from build123d import *

# Parameters (mm, degrees)
BOSS_EXTRUDE1_DEPTH = 10
CUT_EXTRUDE1_START  = -10
CUT_EXTRUDE1_DEPTH  = 10


with BuildPart() as part:
    # Sketch1 → Boss-Extrude1 (new body)
    with BuildSketch(Plane(origin=(0, 0, 0), x_dir=(1, 0, 0), z_dir=(0, 1, 0))):
        Polygon((-19.75, 34.208003449), (-39.5, 0), (-19.75, -34.208003449), (19.75, -34.208003449), (39.5, 0), (19.75, 34.208003449), align=None)
    extrude(amount=BOSS_EXTRUDE1_DEPTH)

    # Sketch7 → Revolve1 (revolve)
    with BuildSketch(Plane(origin=(0, 0, 0), x_dir=(0, 0, -1), z_dir=(1, 0, 0))):
        with BuildLine():
            Line((0, 10), (0, 50))
            Line((0, 50), (3.95, 50))
            Line((3.95, 50), (3.95, 27.320508076))
            ThreePointArc((3.95, 27.320508076), (6.629491924, 17.320508076), (13.95, 10))
            Line((13.95, 10), (0, 10))
        make_face()
    revolve(axis=Axis((0, 10, 0), (0, 1, 0)))

    # Sketch8 → Cut-Extrude1 (cut)
    with BuildSketch(Plane(origin=(0, 50, 0), x_dir=(1, 0, 0), z_dir=(0, 1, 0)).offset(CUT_EXTRUDE1_START)):
        with BuildLine():
            Line((-3.058185737, -2.5), (-3.058185737, 2.5))
            ThreePointArc((-3.058185737, 2.5), (-3.95, 0), (-3.058185737, -2.5))
        make_face()
    extrude(amount=CUT_EXTRUDE1_DEPTH, mode=Mode.SUBTRACT)


solid = part.part
Verification items for the finished model (mm, model axes). A direction names the side the tool comes from. Give positions to 0.01 mm unless a question says otherwise; leave off trailing zeros. Write each loop counter-clockwise with the first axis right and the second up, starting at its lowest first coordinate (ties: lowest second). Pieces come first, ordered by that corner, then holes. Notation, with made-up numbers: M -27,47.25 L 30,47.25 A32 cw 30,85.25 Z; hole C 83.25,-7 d5. An arc over 180 degrees is marked long. Put each result on its own line as item: value. Start each with the question number.
1. Scan lines: line 1 along Y through (x, z) = (23, -9.5); line 2 along X through (y, z) = (6, -27); line 3 along Z through (x, y) = (-31.5, 9.5). Record each from-to range of solid material in increasing order. Write a range as [from, to].
2. Section check C-C (z = 20.5). Record the cut outline in (x, y), and give its area (3 significant figures).
3. Section check D-D (x = 31.5). Record the cut outline in (y, z), and give its area (3 significant figures).
4. Go/stop test with flat-tipped pins: pin 1 Ø10 at (y, z) = (44.5, -4) entering from -X; pin 2 Ø1.5 at (y, z) = (43, 0.5) entering from -X. Record where each tip stops, or that it passes through.
5. Set-up check for faces 4 (the face through (17, 10, 0)), 5 (the face through (-3.058, 45, 0)), 6 (the face through (0, 5, 34.208)): record each of +Z, -Z, +X, -X, +Y, -Y from which the full face is reachable in a straight line by a thin tool's end or side.
6. Section check B-B (x = 0). Record the cut outline in (y, z), and give its area (3 significant figures).
7. Draft check along X on faces 1 (the face through (3.856, 38.501, 0.856)), 2 (the face through (29.763, 4.93, -16.865)), 3 (the face through (-29.49, 4.93, -17.34)). Enter one of: +X half, -X half, draft (parallel to the pull), parting line (faces both ways), or undercut.
8. Section check A-A (y = 9). Record the cut outline in (x, z), and give its area (3 significant figures).
Answer list:
1. line 1: [0, 10]
1. line 2: [-23.91, 23.91]
1. line 3: [-13.86, 13.86]
2. outline: M -27.66,0 L 27.66,0 L 27.66,10 L -27.66,10 Z
2. area: 553 mm2
3. outline: M 0,-13.86 L 10,-13.86 L 10,13.86 L 0,13.86 Z
3. area: 277 mm2
4. pin 1: x = -3.51
4. pin 2: x = -3.06
5. face 4: +Y
5. face 5: +Z, -Z, -X, +Y
5. face 6: +Z, +X, -X, +Y, -Y
6. outline: M 0,-34.21 L 10,-34.21 L 10,-13.95 A20 cw 27.32,-3.95 L 50,-3.95 L 50,3.95 L 27.32,3.95 A20 cw 10,13.95 L 10,34.21 L 0,34.21 Z
6. area: 1,100 mm2
7. face 1: parting line
7. face 2: +X half
7. face 3: -X half
8. outline: M -39.5,0 L -19.75,-34.21 L 19.75,-34.21 L 39.5,0 L 19.75,34.21 L -19.75,34.21 Z
8. area: 4,050 mm2
